The listing builds one solid part. Answer for the finished solid, in the listing's coordinates (mm). A direction names the side the tool comes from. Coordinates: 2 decimals unless noted, no trailing zeros. Order: outer loops, then holes, each group sorted by start corner. A loop starts at its lowest first (then second) coordinate and runs counter-clockwise, first axis right, second up. Notation, with made-up numbers: (-5, 89) - (45, 89) arc R30 cw to (45, 115) - close; hole circle Ø3 at (75.5, -15.75). An arc over 180 degrees is marked (long way). Use one line per item in the form item = value. Start each with the question number.
Item 1: Section D-D, the plane y = 7 is taken. Write down the section's boundary in (x, z).
Item 2: The mould has two halves that part along Y. Classify faces 1 (the flat face through (25, 51, 0)), 2 (the cylindrical face through (51.01, 0.86, 21.1)), 3 (the flat face through (39, 80, 1)): released by +Y, released by -Y, zero draft, split by the parting line, or undercut.
Item 3: Section A-A, the plane x = 15 is taken. Write down the section's boundary in (y, z).
Item 4: Each of these flat-tipped pins is pushed along its axis until it touches: pin 1 Ø0.6 at (x, z) = (26, 1) entering from -Y; pin 2 Ø0.6 at (y, z) = (75.5, 0.5) entering from -X; pin 3 Ø8 at (x, y) = (23, 70) entering from +Z; pin 4 Ø3 at (x, z) = (-0.5, 12) entering from +Y. Where does it stop, or does it pass through?
Item 5: A tool of negligible diameter and unlimited length cuts with its end or side. For faces 4 (the flat face through (24, 90, 1)), 5 (the flat face through (0, 15, 12)), 6 (the flat face through (50, 63, 1)), from which of +Z, -Z, +X, -X, +Y, -Y can it reach the whole face along a straight path? Write none if from no direction.
Item 6: Section B-B, the plane z = 8 is taken. Write down the section's boundary in (x, y), and give its area (3 significant figures).
Item 7: Consider line 1 along Y through (x, z) = (50.6, 16); line 2 along X through (y, z) = (29.5, 3.5); line 3 along Z through (x, y) = (25.5, 69). Determine where each line is inside the solid, lowest interval first. Write a range as [from, to].
Item 8: Section C-C, the plane y = 77.5 is taken. Write down the section's boundary in (x, z), and give its area (3 significant figures).
from build123d import *

# Parameters (mm, degrees)
BOX004_W          = 30
BOX004_H          = 20
BOX004_DEPTH      = 7
BOX003_W          = 30
BOX003_H          = 40
BOX003_DEPTH      = 6
CYLINDER001_R     = 2
CYLINDER001_DEPTH = 59
CYLINDER_R        = 2
CYLINDER_DEPTH    = 59
BOX002_W          = 2
BOX002_H          = 30
BOX002_DEPTH      = 22
FILLET_R          = 1.9
BOX001_W          = 2
BOX001_H          = 30
BOX001_DEPTH      = 22
FILLET001_R       = 1.9
BOX_W             = 50
BOX_H             = 100
BOX_DEPTH         = 2
FILLET002_R       = 0.8
FILLET003_R       = 3
FILLET004_R       = 3
FILLET005_R       = 3
FILLET006_R       = 3


with BuildPart() as cub001:
    # Box004 → Box004 (new body)
    with BuildSketch(Plane(origin=(9, 70, -3), x_dir=(1, 0, 0), z_dir=(0, 0, 1))):
        with Locations((15, 10)):
            Rectangle(BOX004_W, BOX004_H)
    extrude(amount=BOX004_DEPTH)


with BuildPart() as cub:
    # Box003 → Box003 (new body)
    with BuildSketch(Plane(origin=(10, 10, -2), x_dir=(1, 0, 0), z_dir=(0, 0, 1))):
        with Locations((15, 20)):
            Rectangle(BOX003_W, BOX003_H)
    extrude(amount=BOX003_DEPTH)


with BuildPart() as cilindre001:
    # Cylinder001 → Cylinder001 (new body)
    with BuildSketch(Plane(origin=(-4, 23, 13), x_dir=(0, 0, -1), z_dir=(1, 0, 0))):
        Circle(CYLINDER001_R)
    extrude(amount=CYLINDER001_DEPTH)


with BuildPart() as cylinders:
    # Cylinder → Cylinder (new body)
    with BuildSketch(Plane(origin=(-4, 7, 13), x_dir=(0, 0, -1), z_dir=(1, 0, 0))):
        Circle(CYLINDER_R)
    extrude(amount=CYLINDER_DEPTH)

    # Fusion001: union Cilindre001
    add(cilindre001.part)


with BuildPart() as cylinders_1:
    # Fusion001 placement: moved
    add(cylinders.part.moved(Location((0, 0, 3))))


with BuildPart() as fillet_body:
    # Box002 → Box002 (new body)
    with BuildSketch(Plane(origin=(-2, 0, 0), x_dir=(1, 0, 0), z_dir=(0, 0, 1))):
        with Locations((1, 15)):
            Rectangle(BOX002_W, BOX002_H)
    extrude(amount=BOX002_DEPTH)

    # Fillet
    fillet_edges = [fillet_body.edges().sort_by_distance(p)[0] for p in [
        (-2, 15, 0),
    ]]
    fillet(fillet_edges, radius=FILLET_R)


with BuildPart() as fillet001:
    # Box001 → Box001 (new body)
    with BuildSketch(Plane(origin=(50, 0, 0), x_dir=(1, 0, 0), z_dir=(0, 0, 1))):
        with Locations((1, 15)):
            Rectangle(BOX001_W, BOX001_H)
    extrude(amount=BOX001_DEPTH)

    # Fillet001
    fillet001_edges = [fillet001.edges().sort_by_distance(p)[0] for p in [
        (52, 15, 0),
    ]]
    fillet(fillet001_edges, radius=FILLET001_R)


with BuildPart() as obj1:
    # Box → Box (new body)
    with BuildSketch(Plane.XY):
        with Locations((25, 50)):
            Rectangle(BOX_W, BOX_H)
    extrude(amount=BOX_DEPTH)

    # Fusion: union Fillet body, Fillet001
    add(fillet_body.part)
    add(fillet001.part)

    # Fillet002
    fillet002_edges = [obj1.edges().sort_by_distance(p)[0] for p in [
        (0, 15, 2),
        (50, 15, 2),
    ]]
    fillet(fillet002_edges, radius=FILLET002_R)

    # Cut: cut cylinders
    add(cylinders_1.part, mode=Mode.SUBTRACT)

    # Fillet003
    fillet003_edges = [obj1.edges().sort_by_distance(p)[0] for p in [
        (-1, 30, 22),
        (-1, 0, 22),
        (51, 0, 22),
        (51, 30, 22),
    ]]
    fillet(fillet003_edges, radius=FILLET003_R)

    # Fillet004
    fillet004_edges = [obj1.edges().sort_by_distance(p)[0] for p in [
        (0, 100, 1),
        (50, 100, 1),
    ]]
    fillet(fillet004_edges, radius=FILLET004_R)

    # Cut001: cut Cub
    add(cub.part, mode=Mode.SUBTRACT)

    # Fillet005
    fillet005_edges = [obj1.edges().sort_by_distance(p)[0] for p in [
        (40, 10, 1),
        (10, 10, 1),
        (40, 50, 1),
        (10, 50, 1),
    ]]
    fillet(fillet005_edges, radius=FILLET005_R)

    # Cut002: cut Cub001
    add(cub001.part, mode=Mode.SUBTRACT)

    # Fillet006
    fillet006_edges = [obj1.edges().sort_by_distance(p)[0] for p in [
        (39, 70, 1),
        (9, 70, 1),
        (39, 90, 1),
        (9, 90, 1),
    ]]
    fillet(fillet006_edges, radius=FILLET006_R)


solid = obj1.part
Response:
q1.outline = (-2, 1.9) arc R1.9 ccw to (-0.1, 0) - (50.1, 0) arc R1.9 ccw to (52, 1.9) - (52, 14) - (50, 14) - (50, 2.8) arc R0.8 cw to (49.2, 2) - (0.8, 2) arc R0.8 cw to (0, 2.8) - (0, 14) - (-2, 14) - close; (-2, 18) - (0, 18) - (0, 22) - (-2, 22) - close; (50, 18) - (52, 18) - (52, 22) - (50, 22) - close
q2.face_1 = zero draft
q2.face_2 = released by -Y
q2.face_3 = undercut
q3.outline = (0, 0) - (10, 0) - (10, 2) - (0, 2) - close; (50, 0) - (70, 0) - (70, 2) - (50, 2) - close; (90, 0) - (100, 0) - (100, 2) - (90, 2) - close
q4.pin_1 = 0
q4.pin_2 = 0
q4.pin_3 = 2
q4.pin_4 = 30
q5.face_4 = +Z, -Z
q5.face_5 = +Z, +Y, -Y
q5.face_6 = +Z, -Z, +X, +Y
q6.outline = (-2, 0) - (0, 0) - (0, 30) - (-2, 30) - close; (50, 0) - (52, 0) - (52, 30) - (50, 30) - close
q6.area = 120 mm2
q7.line_1 = [0, 5], [9, 21], [25, 30]
q7.line_2 = [-2, 0], [50, 52]
q7.line_3 = [0, 2]
q8.outline = (0, 0) - (9, 0) - (9, 2) - (0, 2) - close; (39, 0) - (50, 0) - (50, 2) - (39, 2) - close
q8.area = 40.0 mm2
